The model under review builds one solid part; all positions refer to its coordinate system, in mm. A direction names the side the tool comes from. Coordinates: 2 decimals unless noted, no trailing zeros. Write each loop counter-clockwise with the first axis right and the second up, starting at its lowest first coordinate (ties: lowest second). Pieces come first, ordered by that corner, then holes.
1) Add section C-C, the plane y = 0. Give the number of separate pieces and of enclosed holes in the cut face, then the cut area to 3 significant figures.
2) Mouldability with a two-part tool opening along Z and no side actions: class faces 1 (the flat face through (0, 15, -18)), 2 (the flat face through (66, 0, 13)), 3 (the flat face through (75, 0, 17)) as released by +Z, released by -Z, zero draft, split by the parting line, or undercut.
3) Machinability: for faces 4 (the flat face through (53, -15, 18)), 5 (the flat face through (-12, 0, 14)), 6 (the flat face through (13, 14.75, -1)), 7 (the flat face through (39, 18.75, 2)), which of the approach directions +Z, -Z, +X, -X, +Y, -Y give a long, thin tool a straight path to every point of the face, cutting with its end or side? Answer none if there is none.
4) For P1, Ø0.8, axis at y = -5, z = -17.5, coming from the +X side; P2, Ø0.8, axis at y = -5.5, z = -18.5, coming from the -X side, all flat-tipped, find the tip position at first contact; note any pin that passes through.
5) Add section A-A, the plane x = -3. State the section outline as (y, z) points, then the cut area to 3 significant figures.
6) For line 1 (X direction, y = -1, z = 16.5); line 2 (Y direction, x = 75, z = 18.55); line 3 (Z direction, x = -10.5, y = 17.5), list the stretches that pass through material, from the lowest coordinate up.
7) Add section B-B, the plane x = -22. State the section outline as (y, z) points, then the cut area to 4 significant figures.
from build123d import *

# Parameters (mm, degrees)
F0_W          = 24
F0_H          = 34
F1_DEPTH      = 18.75
F1_DEPTH_BACK = 18.75
F2_R          = 2.5
F2_W          = 20
F2_H          = 30
F3_DEPTH      = 2.5
F4_DEPTH      = 60
F5_W          = 29.5
F5_H          = 28.5
F6_DEPTH      = 76.15809
F6_DEPTH_BACK = 25


with BuildPart() as f1:
    # F0 (on Front) → F1 (new body, two sides)
    with BuildSketch(Plane.XZ) as f1_sk:
        Polygon((14.5, 19.5), (-14.5, 19.5), (-14.5, -19.5), (14.5, -19.5), (43.5, -19.5), (67.5, -19.5), (67.5, 19.5), (43.5, 19.5), align=None)
        Rectangle(F0_W, F0_H, mode=Mode.SUBTRACT)
        with Locations((26.5, 0)):
            Rectangle(F0_W, F0_H, mode=Mode.SUBTRACT)
        with Locations((53, 0)):
            Rectangle(F0_W, F0_H, mode=Mode.SUBTRACT)
    extrude(amount=F1_DEPTH)
    extrude(f1_sk.sketch, amount=-F1_DEPTH_BACK)

    # F2 (on face) → F3 (join)
    with BuildSketch(Plane.XY.offset(19.5)):
        Polygon((-29.5, 18.75), (-29.5, -18.75), (82.5, -18.75), (82.5, 18.75), (-14.5, 18.75), align=None)
        with Locations((-22, -8.75)):
            Circle(F2_R, mode=Mode.SUBTRACT)
        with Locations((75, -8.75)):
            Circle(F2_R, mode=Mode.SUBTRACT)
        with Locations((-22, 8.75)):
            Circle(F2_R, mode=Mode.SUBTRACT)
        Rectangle(F2_W, F2_H, mode=Mode.SUBTRACT)
        with Locations((26.5, 0)):
            Rectangle(F2_W, F2_H, mode=Mode.SUBTRACT)
        with Locations((53, 0)):
            Rectangle(F2_W, F2_H, mode=Mode.SUBTRACT)
        with Locations((75, 8.75)):
            Circle(F2_R, mode=Mode.SUBTRACT)
    extrude(amount=-F3_DEPTH)

    # F2 (on face) → F4 (cut)
    with BuildSketch(Plane.XY.offset(19.5)):
        Rectangle(F2_W, F2_H)
        with Locations((53, 0)):
            Rectangle(F2_W, F2_H)
        with Locations((26.5, 0)):
            Rectangle(F2_W, F2_H)
    extrude(amount=-F4_DEPTH, mode=Mode.SUBTRACT)

    # F5 (on Right) → F6 (cut, two sides)
    with BuildSketch(Plane.YZ) as f6_sk:
        with Locations((0, -1.25)):
            Rectangle(F5_W, F5_H)
    extrude(amount=F6_DEPTH, mode=Mode.SUBTRACT)
    extrude(f6_sk.sketch, amount=-F6_DEPTH_BACK, mode=Mode.SUBTRACT)


solid = f1.part
Geometry results:
1. separate pieces: 8
1. enclosed holes: 0
1. area: 240 mm2
2. face 1: zero draft
2. face 2: undercut
2. face 3: released by -Z
3. face 4: +Z, -Z
3. face 5: +Y, -Y
3. face 6: +X, -X
3. face 7: +Z, -Z, +X, -X, +Y
4. P1: stops at x = 67.5
4. P2: stops at x = -14.5
5. outline: (-18.75, -19.5) - (-15, -19.5) - (-15, -17) - (-18.75, -17) - close; (-18.75, 17) - (-15, 17) - (-15, 19.5) - (-18.75, 19.5) - close; (15, -19.5) - (18.75, -19.5) - (18.75, -17) - (15, -17) - close; (15, 17) - (18.75, 17) - (18.75, 19.5) - (15, 19.5) - close
5. area: 37.5 mm2
6. line 1: x = -14.5 to -12, 12 to 14.5, 38.5 to 41, 65 to 67.5
6. line 2: y = -18.75 to -11.25, -6.25 to 6.25, 11.25 to 18.75
6. line 3: z = -19.5 to -17, 17 to 19.5
7. outline: (-18.75, 17) - (-11.25, 17) - (-11.25, 19.5) - (-18.75, 19.5) - close; (-6.25, 17) - (6.25, 17) - (6.25, 19.5) - (-6.25, 19.5) - close; (11.25, 17) - (18.75, 17) - (18.75, 19.5) - (11.25, 19.5) - close
7. area: 68.75 mm2
